Autodesk Inventor part; units mm, degrees
ref_plane "YZ Plane" through (0, 0, 0) normal (1, 0, 0) x (0, 1, 0)
ref_plane "XZ Plane" through (0, 0, 0) normal (0, 1, 0) x (-1, 0, 0)
ref_plane "XY Plane" through (0, 0, 0) normal (0, 0, 1) x (1, 0, 0)
sketch "Sketch1" plane through (0, 0, 0) normal (0, 0, 1) x (1, 0, 0)
  line L0 (0, 0) -> (0, 105)
  line L1 (0, 105) -> (10, 105)
  line L2 (10, 105) -> (10, 10)
  line L3 (10, 10) -> (40, 10)
  line L4 (40, 10) -> (40, 0)
  line L5 (40, 0) -> (0, 0)
  dimension "d0" = 105
  dimension "d1" = 10
  dimension "d2" = 95
  dimension "d3" = 30
  dimension "d4" = 10
  dimension "d5" = 40
extrude "Extrusion1" add sketch "Sketch1" along normal blind 80
sketch "Sketch2" plane through (0, 0, 0) normal (-1, 0, 0) x (0, 0, 1)
  circle A0 centre (40, 34) radius 4
  point P0 (0, 0)
  dimension "d8" = 8
extrude "Extrusion2" cut sketch "Sketch2" against normal blind 10
pattern_linear "Rectangular Pattern1" count 2 spacing 42.5 along (0, 1, 0) of "Extrusion2"
sketch "Sketch3" plane through (0, 0, 0) normal (0, -1, 0) x (1, 0, 0)
  circle A0 centre (26, 40) radius 4
  point P0 (0, 0)
  dimension "d14" = 8
extrude "Extrusion3" cut sketch "Sketch3" against normal blind 10
properties part number "AutoCad Part3"
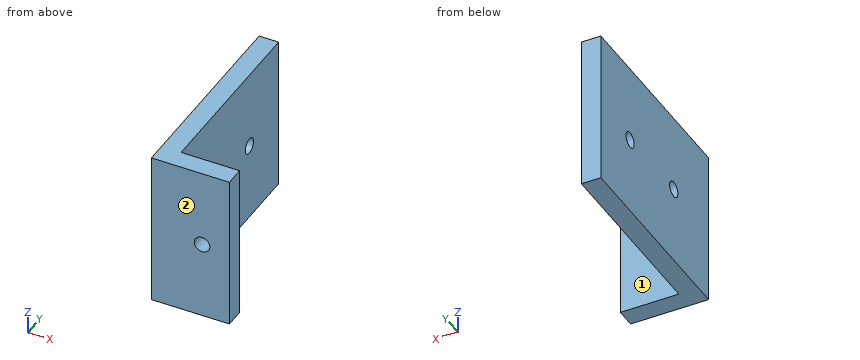
Here's how the part is built. I have some questions about the finished solid (model axes, mm). Face numbers are marked on the shaded views. A direction names the side the tool comes from. Round coordinates to 2 decimals unless told otherwise and drop trailing zeros. Order: outer loops, then holes, each group sorted by start corner. A loop starts at its lowest first (then second) coordinate and runs counter-clockwise, first axis right, second up. Notation, with made-up numbers: M -3,-21.5 L 10,-21.5 A24 cw 10,-9.5 Z; hole C -28,-33 d1. An arc over 180 degrees is marked long. Return JSON: item names as keys, results as strings. Group by question number.
1. Please list where these lines run through material, in increasing order: probe 1 along Y at (x, z) = (29, 52); probe 2 along Z at (x, y) = (3, 76).
2. If we section it at C-C on z = 40: List the corners of the cut face in (x, y) for me.
3. On a 3-axis mill with a long thin cutter (end or side, diameter ignored), from which of +Z, -Z, +X, -X, +Y, -Y can I reach the whole of each face in a straight line? I mean the marked faces 1 and 2. Say none if no direction works.
4. I'm going to push flat-ended pins straight in: pin 1 Ø12 at (y, z) = (65.5, 62) entering from -X; pin 2 Ø13 at (y, z) = (76.5, 40) entering from +X; pin 3 Ø3 at (x, z) = (27, 30.5) entering from +Y. Where does each tip first touch, or does it pass through?
5. If we section it at A-A on x = 26: List the corners of the cut face in (y, z) for me.
6. If we section it at D-D on x = 35: List the corners of the cut face in (y, z) for me, then the cut area to 3 significant figures.
Reply:
{
 "1": {"probe 1": "0 to 10", "probe 2": "0 to 36.03, 43.97 to 80"},
 "2": {"outline": "M 0,0 L 22,0 L 22,10 L 10,10 L 10,30 L 0,30 Z; M 0,38 L 10,38 L 10,72.5 L 0,72.5 Z; M 0,80.5 L 10,80.5 L 10,105 L 0,105 Z; M 30,0 L 40,0 L 40,10 L 30,10 Z"},
 "3": {"face 1": "+Z, -Z, +X, +Y", "face 2": "+Z, -Z, +X, -X, -Y"},
 "4": {"pin 1": "x = 0", "pin 2": "x = 10", "pin 3": "y = 10"},
 "5": {"outline": "M 0,0 L 10,0 L 10,36 L 0,36 Z; M 0,44 L 10,44 L 10,80 L 0,80 Z"},
 "6": {"outline": "M 0,0 L 10,0 L 10,80 L 0,80 Z", "area": "800 mm^2"}
}
